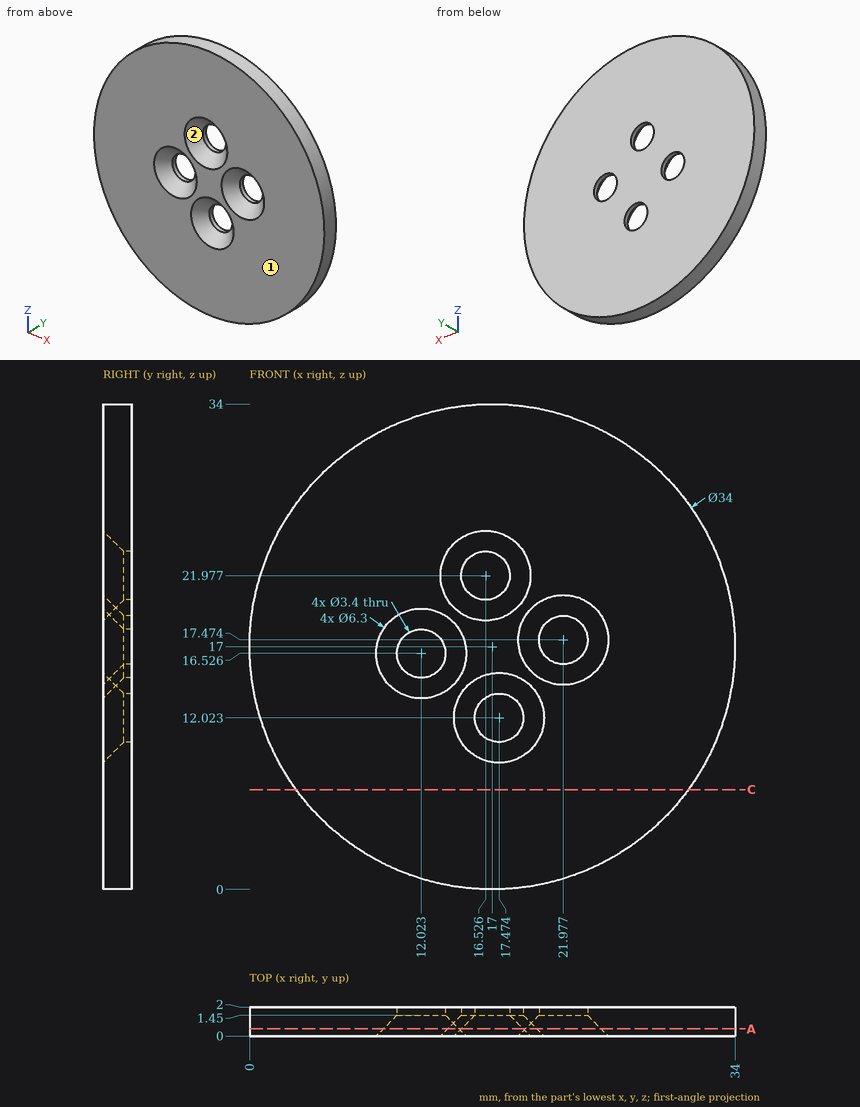
Geometry check sheet. Reference: drawing and pictorial views, mm from the part's lowest x, y, z. Round coordinates to 2 decimals unless told otherwise and drop trailing zeros. Order: outer loops, then holes, each group sorted by start corner. A loop starts at its lowest first (then second) coordinate and runs counter-clockwise, first axis right, second up. Notation, with made-up numbers: (-39, 78.5) - (1, 78.5) arc R13 ccw to (1, 87.5) - close; hole circle Ø9 at (47, 47). An arc over 180 degrees is marked (long way). Use a Markdown table: item, result. Add a question column.
1) Mould release check, pull along Z, two halves, no side actions. Record for the marked faces 1 and 2: released by +Z, released by -Z, zero draft, split by the parting line, or undercut.
2) Section check C-C (z = 7). Record the cut outline in (x, y).
3) Thickness scan on line 1 along X through (y, z) = (1.7, 16) (1 decimal); line 2 along Z through (x, y) = (22.5, 0.2) (1 decimal); line 3 along X through (y, z) = (0.25, 11.5) (1 decimal). Record the ranges inside material, lowest first.
4) Section check A-A (y = 0.5). Count the separate pieces of the cut face and the enclosed holes in it, then the cut area to 3 significant figures.
5) Gauge pin test, flat ends, axial feed: P1, Ø5.5, axis at x = 17.47, z = 12.02, coming from the -Y side (1 decimal); P2, Ø4.5, axis at x = 21.98, z = 17.47, coming from the -Y side (1 decimal); P3, Ø4, axis at x = 19, z = 27.5, coming from the -Y side. Record the tip position at first contact, or that the pin passes through.
Established:
| question | item | result |
|---|---|---|
| 1 | face 1 | zero draft |
| 1 | face 2 | undercut |
| 2 | outline | (3.25, 0) - (30.75, 0) - (30.75, 2) - (3.25, 2) - close |
| 3 | line 1 | 0 to 10.4, 13.6 to 21.1, 22.8 to 34 |
| 3 | line 2 | 0.9 to 14.6, 20.4 to 33.1 |
| 3 | line 3 | 0.9 to 14.6, 20.3 to 33.1 |
| 4 | separate pieces | 1 |
| 4 | enclosed holes | 4 |
| 4 | area | 820 mm2 |
| 5 | P1 | y = 0.4 |
| 5 | P2 | y = 0.9 |
| 5 | P3 | y = 0 |
